```python
from build123d import *

# Parameters (mm, degrees)
BOSS_EXTRUDE1_DEPTH     = 12.5
FILLET1_R               = 10
CUT_EXTRUDE1_DEPTH      = 206.563250607
CUT_EXTRUDE1_DEPTH_BACK = 206.563250607
FILLET5_R               = 10


with BuildPart() as part:
    # Sketch1 → Boss-Extrude1 (new body)
    with BuildSketch(Plane(origin=(0, 0, 0), x_dir=(1, 0, 0), z_dir=(0, 1, 0))):
        Polygon((0, 0), (140, 0), (140, 12.5), (110, 12.5), (110, 150), (30, 150), (30, 12.5), (0, 12.5), align=None)
    extrude(amount=BOSS_EXTRUDE1_DEPTH)

    # Fillet1
    fillet1_edges = [part.edges().sort_by_distance(p)[0] for p in [
        (140, 6.25, 0),
        (0, 6.25, 0),
    ]]
    fillet(fillet1_edges, radius=FILLET1_R)

    # Sketch3 → Cut-Extrude1 (cut, two sides: drawn at the far end of the back side and taken through both)
    with BuildSketch(Plane(origin=(0, 0, 0), x_dir=(0, 0, -1), z_dir=(1, 0, 0)).offset(-CUT_EXTRUDE1_DEPTH_BACK)):
        Polygon((0, 0), (12.5, 12.5), (0, 12.5), align=None)
    extrude(amount=CUT_EXTRUDE1_DEPTH + CUT_EXTRUDE1_DEPTH_BACK, mode=Mode.SUBTRACT)

    # Fillet5
    fillet5_edges = [part.edges().sort_by_distance(p)[0] for p in [
        (30, 6.25, -12.5),
        (110, 6.25, -12.5),
    ]]
    fillet(fillet5_edges, radius=FILLET5_R)


solid = part.part
```
Input: part model. Units: mm. Frame: model coordinates. A direction names the side the tool comes from. Round coordinates to 2 decimals unless told otherwise and drop trailing zeros. Write each loop counter-clockwise with the first axis right and the second up, starting at its lowest first coordinate (ties: lowest second). Pieces come first, ordered by that corner, then holes. Notation, with made-up numbers: M 2.5,0 L 9.5,0 A26 ccw 9.5,28 Z; hole C -33,-28 d8. An arc over 180 degrees is marked long. Write each question's results on one line, items separated by ' | '.
Q1. Line query: line 1 along X through (y, z) = (2.25, -72.5); line 2 along Z through (x, y) = (122, 4.25); line 3 along Z through (x, y) = (27, 3). Output: solid intervals per line, ascending.
Results:
line 1: x = 30 to 110 | line 2: z = -12.5 to -4.25 | line 3: z = -15.36 to -3
Q2. Access query for faces 1 (the face through (30, 6, -87)), 2 (the face through (71, 6, -150)), 3 (the face through (130, 6, -12.5)). Directions: +Z, -Z, +X, -X, +Y, -Y. A direction counts if a zero-diameter tool reaches every point of the face in a straight line with its end or side. Return the directions, or none.
Results:
face 1: -Z, -X, +Y, -Y | face 2: -Z, +X, -X, +Y, -Y | face 3: -Z, +X, +Y, -Y
Q3. Pin query (flat end, axial travel): P1, Ø4, axis at y = 6, z = -69, coming from the -X side; P2, Ø6, axis at x = 30, y = 7.5, coming from the +Z side; P3, Ø1.5, axis at x = 113.5, y = 9, coming from the +Z side. Return the tip coordinate at first contact, or that it passes through.
Results:
P1: stops at x = 30 | P2: stops at z = -4.5 | P3: stops at z = -8.25
Q4. Section query C-C (x = 103). Return loops of the section in (y, z).
Results:
outline: M 0,-150 L 12.5,-150 L 12.5,-12.5 L 0,0 Z
Q5. Section query B-B (z = -102.5). Return loops of the section in (x, y).
Results:
outline: M 30,0 L 110,0 L 110,12.5 L 30,12.5 Z
Q6. Section query A-A (y = 3). Return loops of the section in (x, z), and give its area (3 significant figures).
Results:
outline: M 0,-12.5 L 20,-12.5 A10 cw 30,-22.5 L 30,-150 L 110,-150 L 110,-22.5 A10 cw 120,-12.5 L 140,-12.5 L 140,-10 A10 ccw 137.14,-3 L 2.86,-3 A10 ccw 0,-10 Z | area: 12,400 mm^2
